Read the model definition and answer for the solid it produces. Units are mm, in the model's axes. A direction names the side the tool comes from. Give positions to 0.01 mm unless a question says otherwise; leave off trailing zeros. Order: outer loops, then holes, each group sorted by start corner. A loop starts at its lowest first (then second) coordinate and runs counter-clockwise, first axis right, second up. Notation, with made-up numbers: M -6,23 L 8,23 A29 cw 8,43 Z; hole C 64,-8 d4. An arc over 180 degrees is marked long. Write item = value, one per line. Start each with the question number.
from build123d import *

# Parameters (mm, degrees)
SKETCH_R    = 8
SKETCH_R_2  = 3
PAD_DEPTH   = 10
FILLET_R    = 10
FILLET001_R = 1
FILLET002_R = 2
FILLET003_R = 1
FILLET004_R = 2


with BuildPart() as part:
    # Sketch → Pad (new body)
    with BuildSketch(Plane.XY):
        Polygon((-25, 45), (55, 45), (55, -75), (40, -75), (40, -62.235414), (40, -59), (37.734539, -59), (7.625614, -16), (-25, -16), align=None)
        Circle(SKETCH_R, mode=Mode.SUBTRACT)
        with Locations((40, -52)):
            Circle(SKETCH_R_2, mode=Mode.SUBTRACT)
        with Locations((40, 22)):
            Circle(SKETCH_R_2, mode=Mode.SUBTRACT)
        with Locations((-10, 22)):
            Circle(SKETCH_R_2, mode=Mode.SUBTRACT)
    extrude(amount=PAD_DEPTH)

    # Fillet
    fillet_edges = [part.edges().sort_by_distance(p)[0] for p in [
        (-25, -16, 5),
        (-25, 45, 5),
    ]]
    fillet(fillet_edges, radius=FILLET_R)

    # Fillet001
    fillet001_edges = [part.edges().sort_by_distance(p)[0] for p in [
        (55, -75, 5),
        (40, -75, 5),
        (55, 45, 5),
    ]]
    fillet(fillet001_edges, radius=FILLET001_R)

    # Fillet002
    fillet002_edges = [part.edges().sort_by_distance(p)[0] for p in [
        (40, -59, 5),
    ]]
    fillet(fillet002_edges, radius=FILLET002_R)

    # Fillet003
    fillet003_edges = [part.edges().sort_by_distance(p)[0] for p in [
        (37.734539, -59, 5),
    ]]
    fillet(fillet003_edges, radius=FILLET003_R)

    # Fillet004
    fillet004_edges = [part.edges().sort_by_distance(p)[0] for p in [
        (7.625614, -16, 5),
    ]]
    fillet(fillet004_edges, radius=FILLET004_R)


solid = part.part
1) Each of these flat-tipped pins is pushed along its axis until it touches: P1, Ø2, axis at y = -63, z = 3, coming from the -X side; P2, Ø3, axis at x = 1, z = 7, coming from the -Y side; P3, Ø1.5, axis at y = -42.5, z = 8, coming from the -X side. Where does it stop, or does it pass through?
2) For faces 5 (the face through (40, -67, 5)), 6 (the face through (37.79, -49.97, 4.93)), determine the directions among +Z, -Z, +X, -X, +Y, -Y from which every point of the face is accessible in a straight line to the end or side of a thin tool.
3) For a pull along X with two mould halves and no side action, classify faces 1 (the face through (-25, 14, 5)), 2 (the face through (-12.4, 20.2, 4.9)), 3 (the face through (-1.73, -7.81, 4.93)), 4 (the face through (24, -1, 0)) as pulls with the +X half, pulls with the -X half, needs draft (parallel to the pull), parting line crosses it, or undercut.
4) Find section B-B on x = -10. Determine the outline of the cut face in (y, z).
5) Find section D-D on z = 3.5. Count the separate pieces of the cut face and the enclosed holes in it, plus the area to 3 significant figures.
6) Find the intervals of material crossed by probe 1 along Y at (x, z) = (-10, 4.5); probe 2 along Y at (x, z) = (-0.5, 3); probe 3 along X at (y, z) = (35.5, 9), in increasing order. Write a range as [from, to].
7) Find section C-C on y = 22. Determine the outline of the cut face in (x, z).
8) Find section A-A on y = 0. Determine the outline of the cut face in (x, z).
Numbers:
q1.P1 = 40
q1.P2 = -16
q1.P3 = 25.66
q2.face_5 = +Z, -Z, -X, -Y
q2.face_6 = +Z, -Z
q3.face_1 = pulls with the -X half
q3.face_2 = undercut
q3.face_3 = undercut
q3.face_4 = needs draft
q4.outline = M -16,0 L 19,0 L 19,10 L -16,10 Z; M 25,0 L 45,0 L 45,10 L 25,10 Z
q5.separate_pieces = 1
q5.enclosed_holes = 4
q5.area = 6,180 mm2
q6.probe_1 = [-16, 19], [25, 45]
q6.probe_2 = [-16, -7.98], [7.98, 45]
q6.probe_3 = [-24.99, 55]
q7.outline = M -25,0 L -13,0 L -13,10 L -25,10 Z; M -7,0 L 37,0 L 37,10 L -7,10 Z; M 43,0 L 55,0 L 55,10 L 43,10 Z
q8.outline = M -25,0 L -8,0 L -8,10 L -25,10 Z; M 8,0 L 55,0 L 55,10 L 8,10 Z
